```python
from build123d import *

# Parameters (mm, degrees)
F1_DEPTH    = 6.35
F2_R        = 2.54
F3_R        = 1.905
F4_DEPTH    = 25.4
F5_R        = 3.6608290009
F6_DEPTH    = 1.524
F7_T1_DEPTH = 34.0803226462


# Not quite as in the source:
# - a fillet or chamfer that OpenCascade refuses, or shapes differently, is made with other operations: its cross-section is extruded or revolved along the edge and cut away or added
# - a feature names something its author has since deleted; it is built from what else it names


with BuildPart() as f1:
    # F0 (on Top) → F1 (new body, symmetric)
    with BuildSketch(Plane.XY):
        with BuildLine():
            ThreePointArc((40.64, 0), (-9.9515149654, -39.402753075), (-35.7663459593, 19.2971007335))
            Line((-35.7663459593, 19.2971007335), (-38.5605917374, 20.8046867283))
            Line((-38.5605917374, 20.8046867283), (-38.5605917374, 40.64))
            Line((-38.5605917374, 40.64), (-43.815, 40.64))
            Line((-43.815, 40.64), (-43.815, -43.815))
            Line((-43.815, -43.815), (-43.815, -56.6207952306))
            Line((-43.815, -56.6207952306), (-38.5605917374, -56.6207952306))
            Line((-38.5605917374, -56.6207952306), (-38.5605917374, -43.815))
            Line((-38.5605917374, -43.815), (-38.5605917374, -20.8046867283))
            ThreePointArc((-38.5605917374, -20.8046867283), (10.7289770721, -42.481093159), (43.815, 0))
            Line((43.815, 0), (40.64, 0))
        make_face()
    extrude(amount=F1_DEPTH, both=True)

    # F2
    f2_edges = [f1.edges().sort_by_distance(p)[0] for p in [
        (42.2275, 0, 6.35),
        (42.2275, 0, -6.35),
        (-38.560592, -20.804687, 0),
        (-41.187796, 40.64, 6.35),
        (-41.187796, 40.64, -6.35),
        (-41.187796, -56.620795, 6.35),
        (-41.187796, -56.620795, -6.35),
    ]]
    fillet(f2_edges, radius=F2_R)

    # F3 (on face) → F4 (cut)
    with BuildSketch(Plane(origin=(-43.815, 0, 0), x_dir=(0, -1, 0), z_dir=(-1, 0, 0))):
        with Locations((-30.1695157966, 0)):
            Circle(F3_R)
        with Locations((48.4138801694, 0)):
            Circle(F3_R)
    extrude(amount=-F4_DEPTH, mode=Mode.SUBTRACT)

    # F5 (on face) → F6 (cut)
    with BuildSketch(Plane.YZ.offset(-38.5605917374)):
        with Locations((30.1695157966, 0)):
            Circle(F5_R)
        with Locations((-48.4138801694, 0)):
            Circle(F5_R)
    extrude(amount=-F6_DEPTH, mode=Mode.SUBTRACT)

    # F7: fillet of radius 5.08 on 1 edges, made by hand

    # F7_s2 → F7_t1 (cut)
    with BuildSketch(Plane.XY.offset(-17.0401613231)):
        with BuildLine():
            ThreePointArc((-37.5959569593, 15.4322266804), (-37.2954100255, 18.259021389), (-38.5605917374, 20.8046867283))
            Line((-38.5605917374, 20.8046867283), (-35.7663459593, 19.2971007335))
            ThreePointArc((-35.7663459593, 19.2971007335), (-36.7320185294, 17.3887439097), (-37.5959569593, 15.4322266804))
        make_face()
    extrude(amount=F7_T1_DEPTH, mode=Mode.SUBTRACT)


solid = f1.part
```
Here's how the part is built. I have some questions about the finished solid (model axes, mm). A direction names the side the tool comes from. Coordinates: 2 decimals unless noted, no trailing zeros. Write each loop counter-clockwise with the first axis right and the second up, starting at its lowest first coordinate (ties: lowest second). Pieces come first, ordered by that corner, then holes. Notation, with made-up numbers: (29, -34) - (50, -34) arc R12 ccw to (50, -16) - close; hole circle Ø10 at (43, 33). An arc over 180 degrees is marked (long way). One line per item, written item: value.
1) On a 3-axis mill with a long thin cutter (end or side, diameter ignored), from which of +Z, -Z, +X, -X, +Y, -Y can I reach the whole of each face in a straight line? I mean faces 1 (the flat face through (-41, -56.621, 0)), 2 (the flat face through (-40.085, -47, -2)), 3 (the flat face through (-38.561, 33, -3)), 4 (the flat face through (-41, 40.64, 0)), 5 (the cylindrical face through (42.165, -0.724, -5.586)). Say none if no direction works.
Model answer:
face 1: +Z, -Z, +X, -X, -Y
face 2: +X
face 3: +Z, -Z, +X, +Y
face 4: +Z, -Z, +X, -X, +Y
face 5: -Z, +X, +Y
2) We'd pull the mould along Z, two halves only. Please class faces 6 (the cylindrical face through (-41.2, 39.9, 5.6)), 7 (the cylindrical face through (-39.31, -52.07, 0.16)), 8 (the cylindrical face through (13.915, -41.547, 0.089)), 9 (the flat face through (-29.4, -28.3, -6.35)): pulls with the +Z half, pulls with the -Z half, needs draft (parallel to the pull), parting line crosses it, or undercut.
Model answer:
face 6: pulls with the +Z half
face 7: undercut
face 8: needs draft
face 9: pulls with the -Z half
3) Suppose I cut it at B-B on x = 0. Write out the boundary of the cut face in (y, z) (3 decimals).
Model answer:
outline: (-43.815, -6.35) - (-40.64, -6.35) - (-40.64, 6.35) - (-43.815, 6.35) - close
4) Suppose I cut it at A-A on z = 0. Write out the boundary of the cut face in (x, y) (3 decimals), and give its area (3 significant figures).
Model answer:
outline: (-43.815, -56.621) - (-38.561, -56.621) - (-38.561, -52.075) - (-40.085, -52.075) - (-40.085, -50.319) - (-43.815, -50.319) - close; (-43.815, -46.509) - (-40.085, -46.509) - (-40.085, -44.753) - (-38.561, -44.753) - (-38.561, -29.177) arc R2.54 cw to (-34.047, -27.578) arc R43.815 ccw to (43.815, 0) - (40.64, 0) arc R40.64 cw (long way) to (-37.596, 15.432) arc R5.08 ccw to (-38.561, 20.805) - (-38.561, 26.509) - (-40.085, 26.509) - (-40.085, 28.265) - (-43.815, 28.265) - close; (-43.815, 32.075) - (-40.085, 32.075) - (-40.085, 33.83) - (-38.561, 33.83) - (-38.561, 40.64) - (-43.815, 40.64) - close
area: 809 mm²
5) I'm going to push flat-ended pins straight in: P1, Ø2, axis at x = 31.5, z = -3, coming from the +Y side; P2, Ø3.5, axis at y = -48, z = 1, coming from the +X side; P3, Ø4, axis at y = -37.5, z = 1.5, coming from the +X side. Where does each tip first touch, or does it pass through?
Model answer:
P1: stops at y = -24.4
P2: stops at x = -40.08
P3: stops at x = 25.68
6) Suppose I cut it at C-C on y = 12.5. Write out the boundary of the cut face in (x, z) (3 decimals).
Model answer:
outline: (-43.815, -6.35) - (-38.67, -6.35) - (-38.67, 6.35) - (-43.815, 6.35) - close
7) I need wall thicknesses on line 1 along X through (y, z) = (-32.5, 5.25) (3 decimals); line 2 along X through (y, z) = (-50.5, 1.5) (3 decimals); line 3 along X through (y, z) = (-22.5, -2.25) (3 decimals). Which ranges of each line are inside material? Lowest first, please.
Model answer:
line 1: x = -43.815 to -38.561, -29.385 to -24.4, 24.4 to 29.385
line 2: x = -43.815 to -40.085
line 3: x = -43.815 to -33.843, 33.843 to 37.597
